The listing builds one solid part. Answer for the finished solid, in the listing's coordinates (mm). Face numbers are marked on the shaded views. A direction names the side the tool comes from. Give positions to 0.01 mm unless a question says otherwise; leave off trailing zeros. Loops run counter-clockwise (first coordinate to the right, second up) from the corner with the lowest first, then second, coordinate; pieces in that order, holes last. Notation, with made-up numbers: (43.25, 25.25) - (99.25, 25.25) arc R24 cw to (99.25, 37.25) - close; hole circle Ø4 at (3, -12.5). An arc over 180 degrees is marked (long way). Write each question's results on one line, items separated by ' | '.
from build123d import *


with BuildPart() as part:
    # Sketch1 → Revolve1 (revolve)
    with BuildSketch(Plane(origin=(0, 0, 0), x_dir=(0, 0, -1), z_dir=(1, 0, 0))):
        with BuildLine():
            Line((0, 0), (0, 82.79))
            Line((0, 82.79), (2.5, 82.79))
            Line((2.5, 82.79), (2.5, 78.19))
            Line((2.5, 78.19), (1.5, 78.19))
            Line((1.5, 78.19), (1.5, 75.19))
            Line((1.5, 75.19), (2.5, 75.19))
            Line((2.5, 75.19), (2.5, 14.875520468))
            ThreePointArc((2.5, 14.875520468), (4.566466597, 8.787906178), (9.911809549, 5.216262205))
            Line((9.911809549, 5.216262205), (17.25, 3.25))
            Line((17.25, 3.25), (18.5, 2))
            Line((18.5, 2), (18.5, 1.5))
            ThreePointArc((18.5, 1.5), (9.280355597, 0.375614308), (0, 0))
        make_face()
    revolve(axis=Axis((0, 0, 0), (0, 1, 0)))


solid = part.part
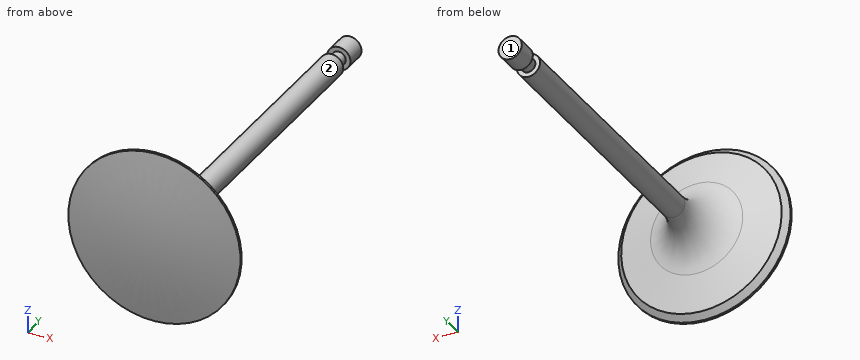
Item 1: Flat-ended cylindrical pins translate along their axes: P1, Ø10, axis at x = -6.5, y = 29.5, coming from the +Z side; P2, Ø5, axis at x = 6.5, z = 9, coming from the -Y side; P3, Ø6, axis at x = -5, y = 38.5, coming from the +Z side. Find the tip coordinate at first contact, or state that the pin passes through.
Values found:
P1: stops at z = 2 | P2: stops at y = 0.32 | P3: stops at z = 1.5
Item 2: A cutting plane is placed at A-A, the plane z = 0. Determine the outline of the cut face in (x, y), plus the area to 3 significant figures.
Values found:
outline: (-18.5, 1.5) arc R114.83 ccw to (18.5, 1.5) - (18.5, 2) - (17.25, 3.25) - (9.91, 5.22) arc R10 cw to (2.5, 14.88) - (2.5, 75.19) - (1.5, 75.19) - (1.5, 78.19) - (2.5, 78.19) - (2.5, 82.79) - (-2.5, 82.79) - (-2.5, 78.19) - (-1.5, 78.19) - (-1.5, 75.19) - (-2.5, 75.19) - (-2.5, 14.88) arc R10 cw to (-9.91, 5.22) - (-17.25, 3.25) - (-18.5, 2) - close | area: 573 mm²
Item 3: A cutting plane is placed at C-C, the plane y = 64.5. Determine the outline of the cut face in (x, z), plus the area to 3 significant figures.
Values found:
outline: circle Ø5 at (0, 0) | area: 19.6 mm²
Item 4: A cutting plane is placed at B-B, the plane x = 0. Determine the outline of the cut face in (y, z), plus the area to 3 significant figures.
Values found:
outline: (1.5, -18.5) - (2, -18.5) - (3.25, -17.25) - (5.22, -9.91) arc R10 cw to (14.88, -2.5) - (75.19, -2.5) - (75.19, -1.5) - (78.19, -1.5) - (78.19, -2.5) - (82.79, -2.5) - (82.79, 2.5) - (78.19, 2.5) - (78.19, 1.5) - (75.19, 1.5) - (75.19, 2.5) - (14.88, 2.5) arc R10 cw to (5.22, 9.91) - (3.25, 17.25) - (2, 18.5) - (1.5, 18.5) arc R114.83 ccw to start | area: 573 mm²
Item 5: Find the intervals of material crossed by line 1 along Z through (x, y) = (0, 31); line 2 along Y through (x, z) = (-10.5, -15); line 3 along Y through (x, z) = (9.5, -8), in increasing order. Write a range as [from, to].
Values found:
line 1: z = [-2.5, 2.5] | line 2: y = [1.47, 2.19] | line 3: y = [0.67, 4.54]
Item 6: For the marked faces 1 and 2, determine the directions among +Z, -Z, +X, -X, +Y, -Y from which every point of the face is accessible in a straight line to the end or side of a thin tool.
Values found:
face 1: +Z, -Z, +X, -X, +Y | face 2: +Y
